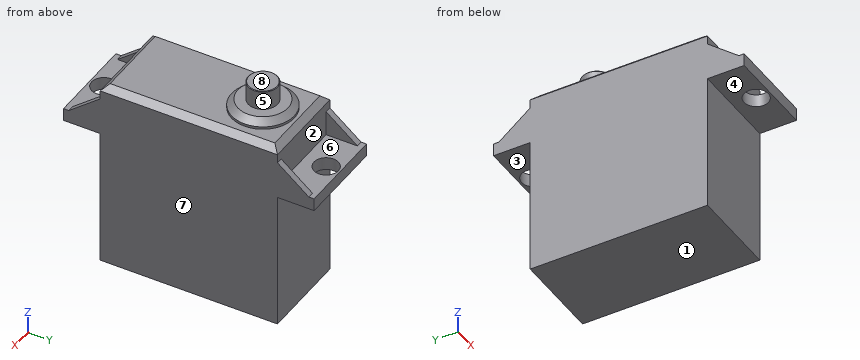
Solid Edge part; units mm, degrees
sketch "Sketch1" plane through (0, 0, 0) normal (0, 0, 1) x (1, 0, 0)
  line L0 (-7.125, -14.15) -> (7.125, -14.15)
  line L1 (7.125, -14.15) -> (7.125, 14.15)
  line L2 (7.125, 14.15) -> (-7.125, 14.15)
  line L3 (-7.125, 14.15) -> (-7.125, -14.15)
  dimension "D1" = 7.125
  dimension "D2" = 7.125
extrude "Protrusion1" add sketch "Sketch1" against normal blind 22.1
sketch "Sketch2" plane through (0, 0, 0) normal (0, 0, 1) x (1, 0, 0)
  line L0 (-7.125, -20) -> (7.125, -20)
  line L1 (7.125, -20) -> (7.125, 20)
  line L2 (7.125, 20) -> (-7.125, 20)
  line L3 (-7.125, 20) -> (-7.125, -20)
  dimension "D1" = 7.125
extrude "ExtrudedProtrusion_2" add sketch "Sketch2" along normal blind 2.05
sketch "Sketch3" plane through (0, 0, 2.05) normal (0, 0, 1) x (1, 0, 0)
  line L0 (7.125, -14.15) -> (-7.125, -14.15)
  line L1 (-7.125, -14.15) -> (-7.125, 14.15)
  line L2 (-7.125, 14.15) -> (7.125, 14.15)
  line L3 (7.125, 14.15) -> (7.125, -14.15)
extrude "ExtrudedProtrusion_3" add sketch "Sketch3" along normal blind 6.4
hole "Hole1" at (0, -17.75, 2.05) direction (0, 0, -1) diameter 3.9 end up to next
hole "Hole2" at (0, 17.75, 2.05) direction (0, 0, -1) diameter 3.9 end up to next
sketch "Sketch4" plane through (0, 0, 8.45) normal (0, 0, 1) x (0, 1, 0)
  circle A0 centre (7.65, 0) radius 2.35
extrude "ExtrudedProtrusion_4" add sketch "Sketch4" along normal blind 4.5
sketch "Sketch5" plane through (0, 0, 8.45) normal (0, 0, 1) x (0, 1, 0)
  circle A0 centre (7.65, 0) radius 5
extrude "ExtrudedProtrusion_5" add sketch "Sketch5" along normal blind 1.4
sketch "Sketch6" plane through (7.125, 0, -6.825) normal (1, 0, 0) x (0, 1, 0)
  line L0 (-14.15, 8.875) -> (-14.15, 12.875)
  line L1 (-14.15, 12.875) -> (-19.15, 8.875)
  line L2 (-19.15, 8.875) -> (-14.15, 8.875)
  line L3 (14.15, 8.875) -> (19.15, 8.875)
  line L4 (19.15, 8.875) -> (14.15, 12.875)
  line L5 (14.15, 12.875) -> (14.15, 8.875)
  dimension "D1" = 14.15
  dimension "D2" = 19.15
extrude "ExtrudedProtrusion_6" add sketch "Sketch6" against normal blind 1
mirror "Mirror1" about plane through (0, 0, 0) normal (1, 0, 0) of "ExtrudedProtrusion_6"
chamfer "Chamfer_1" distance 1 angle 45 4 edges at (-7.125, 0, 8.45) (0, -14.15, 8.45) (7.125, 0, 8.45) (0, 14.15, 8.45)
chamfer "Chamfer_2" distance 1 angle 45 1 edges at (0, 2.65, 9.85)
chamfer "Chamfer_3" distance 0.1 angle 45 1 edges at (0, 5.3, 12.95)
CAD build for the part. Positions are in the model's coordinates, mm. Face numbers are marked on the shaded views. A direction names the side the tool comes from. Coordinates: 2 decimals unless noted, no trailing zeros. Loops run counter-clockwise (first coordinate to the right, second up) from the corner with the lowest first, then second, coordinate; pieces in that order, holes last. Notation, with made-up numbers: (15, 48) - (35, 48) arc R15 cw to (35, 71) - close; hole circle Ø5 at (68, -27.5). An arc over 180 degrees is marked (long way). Return JSON: item names as keys, results as strings.
1. Probe L1, parallel to Y at x = 0, z = 1.6; L2, parallel to X at y = 17.75, z = 0.8 (3 decimals); L3, parallel to Y at x = 1.75, z = -12. List the from-to ranges inside material, lowest first. Write a range as from..to.
Result:
{"L1": "y = -20..-19.7, -15.8..15.8, 19.7..20", "L2": "x = -7.125..-1.95, 1.95..7.125", "L3": "y = -14.15..14.15"}
2. Band-saw the part on B-B (x = 0). State how many separate pieces and enclosed holes the cut face has, and give its area (3 significant figures).
Result:
{"separate pieces": "3", "enclosed holes": "0", "area": "899 mm2"}
3. Mould opens along X. For the marked faces 6, 7 and 8 say: released by +X, released by -X, zero draft, split by the parting line, or undercut.
Result:
{"face 6": "undercut", "face 7": "released by +X", "face 8": "zero draft"}
4. 3-axis set-ups, long thin cutter, end or side, ignore diameter. For the marked faces 1, 2, 3, 4 and 5: which of +Z, -Z, +X, -X, +Y, -Y reach the whole face in a straight line?
Result:
{"face 1": "-Z, +X, -X, +Y, -Y", "face 2": "+Z, +Y", "face 3": "-Z, +X, -X, +Y", "face 4": "-Z, +X, -X, -Y", "face 5": "+Z"}
5. Band-saw the part on C-C (y = 7.65). Give the cut face in (x, z) (3 decimals).
Result:
{"outline": "(-7.125, -22.1) - (7.125, -22.1) - (7.125, 7.45) - (6.125, 8.45) - (5, 8.45) - (5, 8.85) - (4, 9.85) - (2.35, 9.85) - (2.35, 12.85) - (2.25, 12.95) - (-2.25, 12.95) - (-2.35, 12.85) - (-2.35, 9.85) - (-4, 9.85) - (-5, 8.85) - (-5, 8.45) - (-6.125, 8.45) - (-7.125, 7.45) - close"}
6. Band-saw the part on A-A (y = -17.75). Give the cut face in (x, z) (3 decimals).
Result:
{"outline": "(-7.125, 0) - (-1.95, 0) - (-1.95, 2.05) - (-6.125, 2.05) - (-6.125, 3.17) - (-7.125, 3.17) - close; (1.95, 0) - (7.125, 0) - (7.125, 3.17) - (6.125, 3.17) - (6.125, 2.05) - (1.95, 2.05) - close"}
7. Drop flat-ended pins along their axis: pin 1 (1.6 mm diameter, centred on x = -1.5, z = 6, fed in from -Y); pin 2 (3 mm diameter, centred on x = 2, y = -16.5, fed in from +Z); pin 3 (7 mm diameter, centred on x = -3.5, z = -16, fed in from +Y). Give the stop position or say it passes through.
Result:
{"pin 1": "stops at y = -14.15", "pin 2": "stops at z = 2.05", "pin 3": "stops at y = 14.15"}
